Model file for the job. Use its own axes, mm. A direction names the side the tool comes from. Round coordinates to 2 decimals unless told otherwise and drop trailing zeros. Write each loop counter-clockwise with the first axis right and the second up, starting at its lowest first coordinate (ties: lowest second). Pieces come first, ordered by that corner, then holes. Notation, with made-up numbers: (88.5, 36.5) - (122.5, 36.5) arc R25 ccw to (122.5, 56.5) - close; hole circle Ø6 at (64, 3). An arc over 180 degrees is marked (long way). One line per item, written item: value.
from build123d import *

# Parameters (mm, degrees)
CROQUIS1_W              = 50.8
CROQUIS1_H              = 76.2
SALIENTE_EXTRUIR1_DEPTH = 18
CROQUIS2_W              = 50.8
CROQUIS2_H              = 76.2
CROQUIS2_W_2            = 46.12
CROQUIS2_H_2            = 71.52
CROQUIS2_W_3            = 38.8
CROQUIS2_H_3            = 64.2
CORTAR_EXTRUIR1_DEPTH   = 15
CORTAR_EXTRUIR8_DEPTH   = 15
SALIENTE_EXTRUIR3_DEPTH = 41.5
CORTAR_EXTRUIR9_DEPTH   = 51.5
CORTAR_EXTRUIR10_DEPTH  = 51.5
SALIENTE_EXTRUIR4_DEPTH = 16
CORTAR_EXTRUIR11_DEPTH  = 16.5
REDONDEO3_R             = 2
REDONDEO4_R             = 1
CROQUIS15_W             = 48.12
CROQUIS15_H             = 10
CORTAR_EXTRUIR12_DEPTH  = 15
CROQUIS16_W             = 8
CROQUIS16_H             = 1.5
CORTAR_EXTRUIR13_DEPTH  = 2
CROQUIS17_R             = 3
CORTAR_EXTRUIR14_DEPTH  = 10


with BuildPart() as part:
    # Croquis1 → Saliente-Extruir1 (new body)
    with BuildSketch(Plane.XY):
        Rectangle(CROQUIS1_W, CROQUIS1_H)
    extrude(amount=SALIENTE_EXTRUIR1_DEPTH)

    # Croquis2 → Cortar-Extruir1 (cut)
    # profile 1 of 2: a face of its own
    with BuildSketch(Plane.XY.offset(18)):
        Rectangle(CROQUIS2_W, CROQUIS2_H)
        Rectangle(CROQUIS2_W_2, CROQUIS2_H_2, mode=Mode.SUBTRACT)
    # profile 2 of 2: a face of its own
    with BuildSketch(Plane.XY.offset(18)):
        Rectangle(CROQUIS2_W_3, CROQUIS2_H_3)
    extrude(amount=-CORTAR_EXTRUIR1_DEPTH, mode=Mode.SUBTRACT)

    # Croquis6 → Cortar-Extruir8 (cut)
    with BuildSketch(Plane.XY.offset(18)):
        Polygon((-23.06, 35.76), (-8.06, 35.76), (-8.06, 32.1), (-19.4, 32.1), (-19.4, 20.76), (-23.06, 20.76), align=None)
        Polygon((23.06, 35.76), (8.06, 35.76), (8.06, 32.1), (19.4, 32.1), (19.4, 20.76), (23.06, 20.76), align=None)
        Polygon((-23.06, -35.76), (-23.06, -20.76), (-19.4, -20.76), (-19.4, -32.1), (-8.06, -32.1), (-8.06, -35.76), align=None)
        Polygon((23.06, -35.76), (8.06, -35.76), (8.06, -32.1), (19.4, -32.1), (19.4, -20.76), (23.06, -20.76), align=None)
    extrude(amount=-CORTAR_EXTRUIR8_DEPTH, mode=Mode.SUBTRACT)

    # Croquis10 → Saliente-Extruir3 (add)
    with BuildSketch(Plane(origin=(0, -20.76, 0), x_dir=(-1, 0, 0), z_dir=(0, -1, 0))):
        Polygon((23.06, -18), (24.06, -18), (23.06, -3), align=None)
        Polygon((-23.06, -18), (-24.06, -18), (-23.06, -3), align=None)
    extrude(amount=-SALIENTE_EXTRUIR3_DEPTH)

    # Croquis11 → Cortar-Extruir9 (cut)
    with BuildSketch(Plane.XZ.offset(20.76)):
        Polygon((-19.4, 18), (-21.56, 18), (-20.56, 3), (-19.4, 3), align=None)
    extrude(amount=-CORTAR_EXTRUIR9_DEPTH, mode=Mode.SUBTRACT)

    # Croquis12 → Cortar-Extruir10 (cut)
    with BuildSketch(Plane.XZ.offset(20.76)):
        Polygon((19.4, 18), (19.4, 3), (20.56, 3), (21.56, 18), align=None)
    extrude(amount=-CORTAR_EXTRUIR10_DEPTH, mode=Mode.SUBTRACT)

    # Croquis13 → Saliente-Extruir4 (add)
    with BuildSketch(Plane(origin=(8.06, 0, 0), x_dir=(0, 0, -1), z_dir=(1, 0, 0))):
        Polygon((-18, -35.76), (-18, -37.76), (-3, -35.76), align=None)
        Polygon((-18, 35.76), (-18, 37.76), (-3, 35.76), align=None)
    extrude(amount=-SALIENTE_EXTRUIR4_DEPTH)

    # Croquis14 → Cortar-Extruir11 (cut)
    with BuildSketch(Plane(origin=(8.06, 0, 0), x_dir=(0, 0, -1), z_dir=(1, 0, 0))):
        Polygon((-3, -32.1), (-18, -32.1), (-18, -35.26), (-3, -33.26), align=None)
        Polygon((-18, 32.1), (-18, 35.26), (-3, 33.26), (-3, 32.1), align=None)
    extrude(amount=-CORTAR_EXTRUIR11_DEPTH, mode=Mode.SUBTRACT)

    # Redondeo3
    redondeo3_edges = [part.edges().sort_by_distance(p)[0] for p in [
        (-25.4, 38.1, 1.5),
        (25.4, 38.1, 1.5),
        (25.4, -38.1, 1.5),
        (-25.4, -38.1, 1.5),
    ]]
    fillet(redondeo3_edges, radius=REDONDEO3_R)

    # Redondeo4
    redondeo4_edges = [part.edges().sort_by_distance(p)[0] for p in [
        (0, 38.1, 0),
        (-25.4, 0, 0),
        (25.4, 0, 0),
        (0, -38.1, 0),
        (24.814213562, -37.514213562, 0),
        (-24.814213562, -37.514213562, 0),
        (-24.814213562, 37.514213562, 0),
        (24.814213562, 37.514213562, 0),
    ]]
    fillet(redondeo4_edges, radius=REDONDEO4_R)

    # Croquis15 → Cortar-Extruir12 (cut)
    with BuildSketch(Plane.XY.offset(18)):
        with Locations((0, -0.01)):
            Rectangle(CROQUIS15_W, CROQUIS15_H)
    extrude(amount=-CORTAR_EXTRUIR12_DEPTH, mode=Mode.SUBTRACT)

    # Croquis16 → Cortar-Extruir13 (cut)
    with BuildSketch(Plane.XZ.offset(38.1)):
        with Locations((0, 2.25)):
            Rectangle(CROQUIS16_W, CROQUIS16_H)
    extrude(amount=-CORTAR_EXTRUIR13_DEPTH, mode=Mode.SUBTRACT)

    # Croquis17 → Cortar-Extruir14 (cut)
    with BuildSketch(Plane.XY.offset(3)):
        with Locations((13.4, -23.1)):
            Circle(CROQUIS17_R)
        with Locations((13.4, -15.1)):
            Circle(CROQUIS17_R)
        with Locations((5.4, -23.1)):
            Circle(CROQUIS17_R)
    extrude(amount=-CORTAR_EXTRUIR14_DEPTH, mode=Mode.SUBTRACT)


solid = part.part
1. Band-saw the part on C-C on x = 5.4. Write the cut outline in (y, z), plus the area to 3 significant figures.
Report:
outline: (-38.1, 1) arc R1 ccw to (-37.1, 0) - (-26.1, 0) - (-26.1, 3) - (-33.26, 3) - (-35.26, 18) - (-37.76, 18) - (-35.76, 3) - (-38.1, 3) - close; (-20.1, 0) - (37.1, 0) arc R1 ccw to (38.1, 1) - (38.1, 3) - (35.76, 3) - (37.76, 18) - (35.26, 18) - (33.26, 3) - (-20.1, 3) - close
area: 285 mm²
2. Band-saw the part on A-A on y = -23.1. Write the cut outline in (x, z).
Report:
outline: (-25.4, 1) arc R1 ccw to (-24.4, 0) - (2.4, 0) - (2.4, 3) - (-25.4, 3) - close; (8.4, 0) - (10.4, 0) - (10.4, 3) - (8.4, 3) - close; (16.4, 0) - (24.4, 0) arc R1 ccw to (25.4, 1) - (25.4, 3) - (16.4, 3) - close
3. Drop flat-ended pins along their axis: pin 1 (5 mm diameter, centred on x = -17, z = 6.5, fed in from +Y); pin 2 (4 mm diameter, centred on x = -23, z = 11, fed in from +Y); pin 3 (4 mm diameter, centred on y = 9, z = 15, fed in from -X); pin 4 (0.8 mm diameter, centred on x = -2, z = 2.5, fed in from -Y). Give the stop position or say it passes through.
Report:
pin 1: through
pin 2: y = 20.76
pin 3: x = -23.99
pin 4: y = -36.1
4. Tool access for faces 1 (the face through (-4, -37, 2)), 2 (the face through (-23.567, 12.755, 10.605)), 3 (the face through (-22, -5.01, 11)), 4 (the face through (22, 20.76, 11)): list every direction of +Z, -Z, +X, -X, +Y, -Y with a clear straight run to the whole face (end or side of a thin tool).
Report:
face 1: -Y
face 2: -X, +Y, -Y
face 3: +Z, +X, -X
face 4: +Z, +X, -X, +Y
5. Band-saw the part on D-D on z = 17. State how many separate pieces and enclosed holes the cut face has, plus the area to 3 significant figures.
Report:
separate pieces: 6
enclosed holes: 0
area: 238 mm²
6. Mould opens along Z. For faces 5 (the face through (21.053, 12.765, 10.395)), 6 (the face through (23.567, -12.995, 10.605)), 7 (the face through (-8.06, -35, 9)) say: released by +Z, released by -Z, zero draft, split by the parting line, or undercut.
Report:
face 5: released by +Z
face 6: undercut
face 7: zero draft
7. Band-saw the part on B-B on y = -15.1. Write the cut outline in (x, z).
Report:
outline: (-25.4, 1) arc R1 ccw to (-24.4, 0) - (10.4, 0) - (10.4, 3) - (-20.56, 3) - (-21.56, 18) - (-24.06, 18) - (-23.06, 3) - (-25.4, 3) - close; (16.4, 0) - (24.4, 0) arc R1 ccw to (25.4, 1) - (25.4, 3) - (23.06, 3) - (24.06, 18) - (21.56, 18) - (20.56, 3) - (16.4, 3) - close
8. Wall check: probe 1 along Y at (x, z) = (13.4, 2.4); probe 2 along Y at (x, z) = (5.4, 0.95); probe 3 along Z at (x, y) = (-17.5, -33). Give the ranges that are in metal, low to high. Write a range as [from, to].
Report:
probe 1: [-38.1, -26.1], [-20.1, -18.1], [-12.1, 38.1]
probe 2: [-38.1, -26.1], [-20.1, 38.1]
probe 3: [0, 3]
